from build123d import *

# Parameters (mm, degrees)
F1_W      = 152.4
F1_H      = 50.8
F2_DEPTH  = 76.2
F3_W      = 25.4
F3_H      = 38.1
F4_DEPTH  = 76.201
F5_W      = 25.4
F5_H      = 38.1
F6_DEPTH  = 76.201
F9_DEPTH  = 12.701
F11_DEPTH = 127.001


with BuildPart() as f2:
    # F1 (on face) → F2 (new body)
    with BuildSketch(Plane.XZ):
        with Locations((-8.853449, 22.809748)):
            Rectangle(F1_W, F1_H)
    extrude(amount=F2_DEPTH)

    # F3 (on face) → F4 (cut, through all)
    with BuildSketch(Plane.XZ.offset(76.2)):
        with Locations((-72.353449, 29.159748)):
            Rectangle(F3_W, F3_H)
    extrude(amount=-F4_DEPTH, mode=Mode.SUBTRACT)

    # F5 (on face) → F6 (cut, through all)
    with BuildSketch(Plane.XZ.offset(76.2)):
        with Locations((54.646551, 29.159748)):
            Rectangle(F5_W, F5_H)
    extrude(amount=-F6_DEPTH, mode=Mode.SUBTRACT)

    # F8 (on face) → F9 (cut, through all)
    with BuildSketch(Plane.XY.offset(10.109748)):
        Polygon((41.946551, -50.8), (67.346551, -76.2), (67.346551, 0), (41.946551, -25.4), align=None)
        Polygon((67.346551, 0), (67.346551, -76.2), (78.186899, -95.031939), (78.186899, -19.507643), align=None)
    extrude(amount=-F9_DEPTH, mode=Mode.SUBTRACT)

    # F10 (on face) → F11 (cut, through all)
    with BuildSketch(Plane.YZ.offset(41.946551)):
        Polygon((-25.4, 48.209748), (-50.8, 48.209748), (-38.1, 35.509748), align=None)
    extrude(amount=-F11_DEPTH, mode=Mode.SUBTRACT)


solid = f2.part
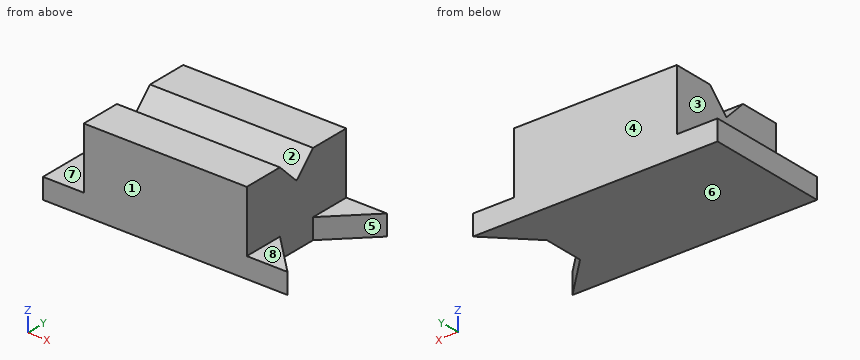
Can you work these out from the model? Positions are in its coordinate system, mm. Face numbers are marked on the shaded views. A direction names the side the tool comes from. Round coordinates to 2 decimals unless told otherwise and drop trailing zeros. Write each loop counter-clockwise with the first axis right and the second up, starting at its lowest first coordinate (ties: lowest second). Pieces come first, ordered by that corner, then holes. Notation, with made-up numbers: (31.5, -10) -> (85.5, -10) arc R22 cw to (85.5, 0) -> close; hole circle Ø7 at (51, 20). An arc over 180 degrees is marked (long way). One line per question, with ' | ' between items. Start each with the question number.
1) I need wall thicknesses on line 1 (X direction, y = -21.5, z = 44); line 2 (X direction, y = -37.5, z = 10); line 3 (Y direction, x = 59.5, z = 4). Which ranges of each line are inside material? Lowest first, please. Write a range as [from, to].
2) Suppose I cut it at A-A on x = 16.5. Write out the boundary of the cut face in (y, z), then the cut area to 3 significant figures.
3) Suppose I cut it at D-D on z = 33. Write out the boundary of the cut face in (x, y).
4) I'm going to push flat-ended pins straight in: P1, Ø7.5, axis at x = 56.5, y = -10, coming from the +Z side; P2, Ø19, axis at y = -43.5, z = 31.5, coming from the -X side; P3, Ø15, axis at y = -39.5, z = 31, coming from the +X side. Where does each tip first touch, or does it pass through?
5) Suppose I cut it at C-C on x = 49. Write out the boundary of the cut face in (y, z).
6) On a 3-axis mill with a long thin cutter (end or side, diameter ignored), from which of +Z, -Z, +X, -X, +Y, -Y can I reach the whole of each face in a straight line? I mean the marked faces 5, 6, 7 and 8. Say none if no direction works.
7) Suppose I cut it at B-B on y = -57. Write out the boundary of the cut face in (x, z), then the cut area to 3 significant figures.
8) If we mould it in two halves opening along Y, with no side actions, what happens to the marked faces 1, 2, 3 and 4? For each: released by +Y, released by -Y, zero draft, split by the parting line, or undercut.
Return value:
1) line 1: x = [-59.65, 41.95] | line 2: x = [-85.05, 41.95] | line 3: y = [-76.2, -68.35], [-7.85, 0]
2) outline: (-76.2, -2.59) -> (0, -2.59) -> (0, 48.21) -> (-25.4, 48.21) -> (-38.1, 35.51) -> (-50.8, 48.21) -> (-76.2, 48.21) -> close | area: 3,710 mm2
3) outline: (-59.65, -76.2) -> (41.95, -76.2) -> (41.95, 0) -> (-59.65, 0) -> close
4) P1: stops at z = 10.11 | P2: stops at x = -59.65 | P3: stops at x = 41.95
5) outline: (-76.2, -2.59) -> (-57.85, -2.59) -> (-57.85, 10.11) -> (-76.2, 10.11) -> close; (-18.35, -2.59) -> (0, -2.59) -> (0, 10.11) -> (-18.35, 10.11) -> close
6) face 5: +Z, -Z, +X | face 6: -Z, +X, -X, +Y, -Y | face 7: +Z, -X, +Y, -Y | face 8: +Z, +X, +Y, -Y
7) outline: (-85.05, -2.59) -> (48.15, -2.59) -> (48.15, 10.11) -> (41.95, 10.11) -> (41.95, 48.21) -> (-59.65, 48.21) -> (-59.65, 10.11) -> (-85.05, 10.11) -> close | area: 5,560 mm2
8) face 1: released by -Y | face 2: undercut | face 3: zero draft | face 4: released by +Y
